from build123d import *

# Parameters (mm, degrees)
F1_DEPTH = 25.4
F2_SIZE  = 1.27


with BuildPart() as f1:
    # F0 (on Top) → F1 (new body)
    with BuildSketch(Plane.XY):
        with BuildLine():
            ThreePointArc((-69.19944, 18.047227), (-73.689569, 19.907098), (-75.54944, 24.397227))
            Line((-75.54944, 24.397227), (-75.54944, 33.922227))
            ThreePointArc((-75.54944, 33.922227), (-73.689569, 38.412355), (-69.19944, 40.272227))
            Line((-69.19944, 40.272227), (-32.523775, 40.272227))
            ThreePointArc((-32.523775, 40.272227), (-29.732398, 39.625797), (-27.509345, 37.81812))
            ThreePointArc((-27.509345, 37.81812), (-20.757849, 38.513879), (-24.350649, 44.272227))
            Line((-24.350649, 44.272227), (-69.359149, 44.272227))
            ThreePointArc((-69.359149, 44.272227), (-72.441141, 45.070306), (-74.748433, 47.263936))
            ThreePointArc((-74.748433, 47.263936), (-83.54944, 48.272227), (-82.54115, 39.471219))
            ThreePointArc((-82.54115, 39.471219), (-80.34752, 37.163927), (-79.54944, 34.081935))
            Line((-79.54944, 34.081935), (-79.54944, 24.237518))
            ThreePointArc((-79.54944, 24.237518), (-80.34752, 21.155526), (-82.54115, 18.848234))
            ThreePointArc((-82.54115, 18.848234), (-83.54944, 10.047227), (-74.748433, 11.055517))
            ThreePointArc((-74.748433, 11.055517), (-72.441141, 13.249147), (-69.359149, 14.047227))
            Line((-69.359149, 14.047227), (-24.350649, 14.047227))
            ThreePointArc((-24.350649, 14.047227), (-20.757849, 19.805574), (-27.509345, 20.501333))
            ThreePointArc((-27.509345, 20.501333), (-29.732398, 18.693656), (-32.523775, 18.047227))
            Line((-32.523775, 18.047227), (-69.19944, 18.047227))
        make_face()
    extrude(amount=F1_DEPTH)

    # F2
    f2_edges = [f1.edges().sort_by_distance(p)[0] for p in [
        (-79.54944, 29.159727, 25.4),
        (-80.34752, 21.155526, 25.4),
        (-50.861608, 40.272227, 25.4),
        (-46.854899, 44.272227, 25.4),
        (-50.861608, 18.047227, 25.4),
        (-83.54944, 10.047227, 25.4),
        (-83.54944, 48.272227, 0),
        (-83.54944, 10.047227, 0),
        (-79.54944, 29.159727, 0),
        (-82.54115, 39.471219, 12.7),
        (-80.34752, 21.155526, 0),
        (-24.350649, 44.272227, 12.7),
        (-29.732398, 18.693656, 25.4),
        (-20.757849, 19.805574, 25.4),
        (-83.54944, 48.272227, 25.4),
        (-79.54944, 24.237518, 12.7),
        (-79.54944, 34.081935, 12.7),
        (-75.54944, 29.159727, 25.4),
        (-82.54115, 18.848234, 12.7),
        (-73.689569, 38.412355, 25.4),
        (-46.854899, 14.047227, 25.4),
        (-32.523775, 18.047227, 12.7),
        (-80.34752, 37.163927, 25.4),
        (-72.441141, 45.070306, 25.4),
        (-73.689569, 19.907098, 25.4),
        (-72.441141, 45.070306, 0),
        (-46.854899, 44.272227, 0),
        (-72.441141, 13.249147, 25.4),
        (-29.732398, 18.693656, 0),
        (-20.757849, 19.805574, 0),
        (-20.757849, 38.513879, 0),
        (-75.54944, 29.159727, 0),
        (-73.689569, 38.412355, 0),
        (-27.509345, 37.81812, 12.7),
        (-69.19944, 18.047227, 12.7),
        (-24.350649, 14.047227, 12.7),
        (-69.359149, 14.047227, 12.7),
        (-75.54944, 24.397227, 12.7),
        (-75.54944, 33.922227, 12.7),
        (-74.748433, 47.263936, 12.7),
        (-69.359149, 44.272227, 12.7),
        (-80.34752, 37.163927, 0),
        (-32.523775, 40.272227, 12.7),
        (-69.19944, 40.272227, 12.7),
        (-73.689569, 19.907098, 0),
        (-50.861608, 18.047227, 0),
        (-29.732398, 39.625797, 25.4),
        (-20.757849, 38.513879, 25.4),
        (-74.748433, 11.055517, 12.7),
        (-27.509345, 20.501333, 12.7),
        (-29.732398, 39.625797, 0),
        (-46.854899, 14.047227, 0),
        (-72.441141, 13.249147, 0),
        (-50.861608, 40.272227, 0),
    ]]
    chamfer(f2_edges, length=F2_SIZE)


solid = f1.part
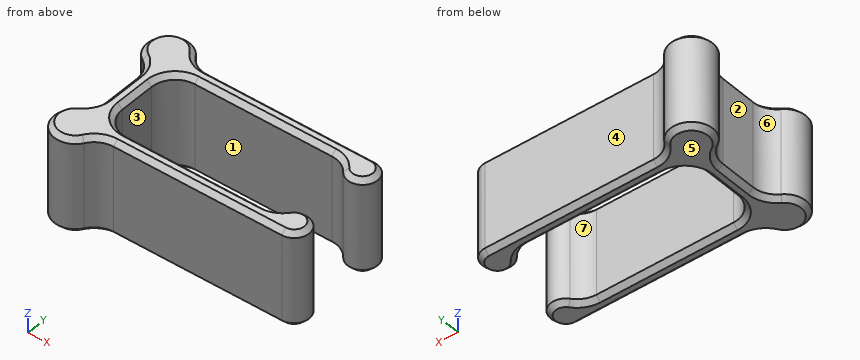
Here's how the part is built. I have some questions about the finished solid (model axes, mm). Face numbers are marked on the shaded views. A direction names the side the tool comes from. Give positions to 0.01 mm unless a question says otherwise; leave off trailing zeros. Order: outer loops, then holes, each group sorted by start corner. A loop starts at its lowest first (then second) coordinate and runs counter-clockwise, first axis right, second up. Notation, with made-up numbers: (73, -11) -> (110, -11) arc R21 cw to (110, -3) -> close; hole circle Ø9 at (29, -5). An arc over 180 degrees is marked (long way). Use a Markdown table: item, result. Add a question column.
Item 1: Imagine slicing it at B-B on y = 31. Please give me the cut outline in (x, z).
Item 2: I need wall thicknesses on line 1 (Y direction, x = -69, z = 4.5); line 2 (X direction, y = 41, z = 13.75). Which ranges of each line are inside material? Lowest first, please.
Item 3: For the marked faces 1, 2 and 3, which set-ups out of +Z, -Z, +X, -X, +Y, -Y let a thin tool reach every point of the face, with its end or its side?
Item 4: If we mould it in two halves opening along Y, with no side actions, what happens to the marked faces 4, 5, 6 and 7? For each: pulls with the +Y half, pulls with the -Y half, needs draft (parallel to the pull), parting line crosses it, or undercut.
Item 5: Imagine slicing it at A-A on x = -36.5. Please give me the cut outline in (y, z), plus the area to 3 significant figures.
Item 6: Will these pins go through, and if not, where does the flat tip stop? pin 1 (4 mm diameter, centred on x = -49, z = 6.5, fed in from +Y); pin 2 (2 mm diameter, centred on x = -49, y = 45.5, fed in from +Z); pin 3 (2 mm diameter, centred on x = -75.5, z = 3, fed in from +Y); pin 4 (5 mm diameter, centred on y = 36.5, z = 7.5, fed in from +X).
Item 7: Imagine slicing it at C-C on z = 4.75. Please give me the cut outline in (x, y).
Data:
| question | item | result |
|---|---|---|
| 1 | outline | (-79.55, 1.27) -> (-78.28, 0) -> (-76.82, 0) -> (-75.55, 1.27) -> (-75.55, 24.13) -> (-76.82, 25.4) -> (-78.28, 25.4) -> (-79.55, 24.13) -> close |
| 2 | line 1 | y = 14.05 to 18.05, 40.27 to 44.27 |
| 2 | line 2 | x = -84.16 to -20.42 |
| 3 | face 1 | +Z, -Z |
| 3 | face 2 | +Z, -Z, -X |
| 3 | face 3 | +Z, -Z, +X |
| 4 | face 4 | pulls with the +Y half |
| 4 | face 5 | needs draft |
| 4 | face 6 | undercut |
| 4 | face 7 | undercut |
| 5 | outline | (14.05, 1.27) -> (15.32, 0) -> (16.78, 0) -> (18.05, 1.27) -> (18.05, 24.13) -> (16.78, 25.4) -> (15.32, 25.4) -> (14.05, 24.13) -> close; (40.27, 1.27) -> (41.54, 0) -> (43, 0) -> (44.27, 1.27) -> (44.27, 24.13) -> (43, 25.4) -> (41.54, 25.4) -> (40.27, 24.13) -> close |
| 5 | area | 197 mm² |
| 6 | pin 1 | stops at y = 44.27 |
| 6 | pin 2 | passes through |
| 6 | pin 3 | stops at y = 49.04 |
| 6 | pin 4 | stops at x = -20.56 |
| 7 | outline | (-82.54, 18.85) arc R5.66 ccw (long way) to (-74.75, 11.06) arc R6.35 cw to (-69.36, 14.05) -> (-24.35, 14.05) arc R4 ccw (long way) to (-27.51, 20.5) arc R6.35 cw to (-32.52, 18.05) -> (-69.2, 18.05) arc R6.35 cw to (-75.55, 24.4) -> (-75.55, 33.92) arc R6.35 cw to (-69.2, 40.27) -> (-32.52, 40.27) arc R6.35 cw to (-27.51, 37.82) arc R4 ccw (long way) to (-24.35, 44.27) -> (-69.36, 44.27) arc R6.35 cw to (-74.75, 47.26) arc R5.66 ccw (long way) to (-82.54, 39.47) arc R6.35 cw to (-79.55, 34.08) -> (-79.55, 24.24) arc R6.35 cw to start |
